Geometry: final body of the model. Coordinates: model frame, mm. A direction names the side the tool comes from. Coordinates: 2 decimals unless noted, no trailing zeros. Write each loop counter-clockwise with the first axis right and the second up, starting at its lowest first coordinate (ties: lowest second). Pieces come first, ordered by that corner, then holes. Notation, with made-up numbers: (26.5, -11.5) - (50.5, -11.5) arc R16 ccw to (50.5, 7.5) - close; hole circle Ø5 at (64, 88). An arc over 180 degrees is marked (long way). Answer as a JSON object with one key per item and string values. Group by question number.
Item 1: First-contact query: pin 1 Ø10 at (x, y) = (19.5, -27) entering from -Z; pin 2 Ø4 at (x, z) = (26, -11.5) entering from +Y; pin 3 Ø3.5 at (x, y) = (-1.5, -3) entering from -Z. Flat tips, straight axial feed; report the tip coordinate or a pass-through.
Item 2: Section B-B on x = 22. Return loops of the section in (y, z), and give its area (3 significant figures).
Item 3: Line query: line 1 along Y through (x, z) = (17, -10.5); line 2 along Z through (x, y) = (17, -31.2); line 3 along X through (y, z) = (-30.05, 6). Output: solid intervals per line, ascending. Write a range as from..to.
Item 4: Section A-A on z = -18. State how many separate pieces and enclosed holes the cut face has, and give its area (3 significant figures).
Item 5: Set-up query: faces 5 (the flat face through (0, -27, 4)), 6 (the cylindrical face through (43.53, -30.48, 0.18)), 7 (the flat face through (13, -19, -7)). Return all of +Z, -Z, +X, -X, +Y, -Y with unobstructed straight access to the full face (end or side cutting, diameter ignored); none if empty.
Item 6: Section D-D on y = -24. Return loops of the section in (x, z), and give its area (4 significant figures).
Item 7: Mould query, pull axis Z, two halves, no side actions, for faces 1 (the cylindrical face through (15.265, -30.479, 5.772)), 2 (the flat face through (22, -5, -3)), 3 (the flat face through (9, -16, -24)), 4 (the flat face through (11, -12, 10)). Classes: pulls with the +Z half, pulls with the -Z half, needs draft (parallel to the pull), parting line crosses it, or undercut.
```python
from build123d import *

# Parameters (mm, degrees)
SZKIC1_W                     = 12
SZKIC1_H                     = 18
SZKIC1_R                     = 1.75
DODANIE_WYCI_GNI_CIE1_DEPTH  = 5
SZKIC2_W                     = 12
SZKIC2_H                     = 36
SZKIC2_R                     = 1.75
DODANIE_WYCI_GNI_CIE2_DEPTH  = 5
SZKIC5_W                     = 34
SZKIC5_H                     = 4
DODANIE_WYCI_GNI_CIE5_DEPTH  = 38
SZKIC6_W                     = 7
SZKIC6_H                     = 34
DODANIE_WYCI_GNI_CIE6_DEPTH  = 18
SZKIC7_R                     = 1.75
WYTNIJ_WYCI_GNI_CIE1_DEPTH   = 4
WYTNIJ_WYCI_GNI_CIE2_DEPTH   = 4
ZAOKR_GLENIE1_R              = 5
SZKIC9_W                     = 5
SZKIC9_H                     = 18
DODANIE_WYCI_GNI_CIE7_DEPTH  = 12
DODANIE_WYCI_GNI_CIE8_DEPTH  = 18
SZKIC11_W                    = 4
SZKIC11_H                    = 34
DODANIE_WYCI_GNI_CIE9_DEPTH  = 2
SZKIC12_R                    = 1.75
SZKIC12_W                    = 4
SZKIC12_H                    = 34
DODANIE_WYCI_GNI_CIE10_DEPTH = 3
SFAZOWANIE1_SIZE             = 3
SFAZOWANIE2_SIZE             = 2
SZKIC13_W                    = 3
SZKIC13_H                    = 34
DODANIE_WYCI_GNI_CIE11_DEPTH = 14
SZKIC14_R                    = 1.75
WYTNIJ_WYCI_GNI_CIE3_DEPTH   = 3


with BuildPart() as part:
    # Szkic1 → Dodanie-wyciągnięcie1 (new body)
    with BuildSketch(Plane.XY):
        Rectangle(SZKIC1_W, SZKIC1_H)
        with Locations((-2, 5)):
            Circle(SZKIC1_R, mode=Mode.SUBTRACT)
        with Locations((2, -5)):
            Circle(SZKIC1_R, mode=Mode.SUBTRACT)
    extrude(amount=DODANIE_WYCI_GNI_CIE1_DEPTH)

    # Szkic2 → Dodanie-wyciągnięcie2 (add)
    with BuildSketch(Plane.XY.offset(5)):
        with Locations((0, -9)):
            Rectangle(SZKIC2_W, SZKIC2_H)
        with Locations((-2, 5)):
            Circle(SZKIC2_R, mode=Mode.SUBTRACT)
        with Locations((2, -5)):
            Circle(SZKIC2_R, mode=Mode.SUBTRACT)
    extrude(amount=DODANIE_WYCI_GNI_CIE2_DEPTH)

    # Szkic5 → Dodanie-wyciągnięcie5 (add)
    with BuildSketch(Plane(origin=(6, 0, 0), x_dir=(0, 0, -1), z_dir=(1, 0, 0))):
        with Locations((7, -7)):
            Rectangle(SZKIC5_W, SZKIC5_H)
    extrude(amount=DODANIE_WYCI_GNI_CIE5_DEPTH)

    # Szkic6 → Dodanie-wyciągnięcie6 (add)
    with BuildSketch(Plane.XZ.offset(9)):
        with Locations((9.5, -7)):
            Rectangle(SZKIC6_W, SZKIC6_H)
    extrude(amount=DODANIE_WYCI_GNI_CIE6_DEPTH)

    # Szkic7 → Wytnij-wyciągnięcie1 (cut)
    with BuildSketch(Plane(origin=(0, -5, 0), x_dir=(1, 0, 0), z_dir=(0, 1, 0))):
        with Locations(Location((17, -6, 0), (0, 0, 270))):
            Circle(SZKIC7_R)
        with Locations(Location((17, 18, 0), (0, 0, 270))):
            Circle(SZKIC7_R)
        with Locations(Location((38.7, -6, 0), (0, 0, 270))):
            Circle(SZKIC7_R)
    extrude(amount=-WYTNIJ_WYCI_GNI_CIE1_DEPTH, mode=Mode.SUBTRACT)

    # Szkic8 → Wytnij-wyciągnięcie2 (cut)
    with BuildSketch(Plane(origin=(0, -5, 0), x_dir=(1, 0, 0), z_dir=(0, 1, 0))):
        Polygon((44, 24), (16, 24), (44, 0), align=None)
    extrude(amount=-WYTNIJ_WYCI_GNI_CIE2_DEPTH, mode=Mode.SUBTRACT)

    # Zaokrąglenie1
    zaokr_glenie1_edges = [part.edges().sort_by_distance(p)[0] for p in [
        (44, -7, 10),
        (16, -7, -24),
        (44, -7, 0),
    ]]
    fillet(zaokr_glenie1_edges, radius=ZAOKR_GLENIE1_R)

    # Szkic9 → Dodanie-wyciągnięcie7 (add)
    with BuildSketch(Plane.ZY.offset(-6)):
        with Locations((2.5, -18)):
            Rectangle(SZKIC9_W, SZKIC9_H)
    extrude(amount=DODANIE_WYCI_GNI_CIE7_DEPTH)

    # Szkic10 → Dodanie-wyciągnięcie8 (add)
    with BuildSketch(Plane.XZ.offset(27)):
        Polygon((6, 0), (1, 0), (6, -5), align=None)
    extrude(amount=-DODANIE_WYCI_GNI_CIE8_DEPTH)

    # Szkic11 → Dodanie-wyciągnięcie9 (add)
    with BuildSketch(Plane.XZ.offset(27)):
        with Locations((11, -7)):
            Rectangle(SZKIC11_W, SZKIC11_H)
    extrude(amount=DODANIE_WYCI_GNI_CIE9_DEPTH)

    # Szkic12 → Dodanie-wyciągnięcie10 (add)
    # profile 1 of 2: a face of its own
    with BuildSketch(Plane.XZ.offset(29)):
        with BuildLine():
            Line((44, 2.299674612), (44, 5))
            ThreePointArc((44, 5), (42.535533906, 8.535533906), (39, 10))
            Line((39, 10), (13, 10))
            Line((13, 10), (13, -24))
            Line((13, -24), (14.150379619, -24))
            ThreePointArc((14.150379619, -24), (15.885110858, -23.689425075), (17.404336486, -22.796283012))
            Line((17.404336486, -22.796283012), (42.253956867, -1.496608399))
            ThreePointArc((42.253956867, -1.496608399), (43.542564492, 0.210390565), (44, 2.299674612))
        make_face()
        with Locations(Location((38.7, 6, 0), (0, 0, 90))):
            Circle(SZKIC12_R, mode=Mode.SUBTRACT)
        with Locations(Location((17, -18, 0), (0, 0, 90))):
            Circle(SZKIC12_R, mode=Mode.SUBTRACT)
        with Locations(Location((17, 6, 0), (0, 0, 90))):
            Circle(SZKIC12_R, mode=Mode.SUBTRACT)
    # profile 2 of 2: a face of its own
    with BuildSketch(Plane.XZ.offset(29)):
        with Locations((11, -7)):
            Rectangle(SZKIC12_W, SZKIC12_H)
    extrude(amount=DODANIE_WYCI_GNI_CIE10_DEPTH)

    # Sfazowanie1
    sfazowanie1_edges = [part.edges().sort_by_distance(p)[0] for p in [
        (9, -27, -7),
    ]]
    chamfer(sfazowanie1_edges, length=SFAZOWANIE1_SIZE)

    # Sfazowanie2
    sfazowanie2_edges = [part.edges().sort_by_distance(p)[0] for p in [
        (9, -32, -7),
    ]]
    chamfer(sfazowanie2_edges, length=SFAZOWANIE2_SIZE - 0.0001)  # a hair under: the kernel refuses the full size

    # Szkic13 → Dodanie-wyciągnięcie11 (add)
    with BuildSketch(Plane(origin=(0, -5, 0), x_dir=(1, 0, 0), z_dir=(0, 1, 0))):
        with Locations((7.5, 7)):
            Rectangle(SZKIC13_W, SZKIC13_H)
    extrude(amount=DODANIE_WYCI_GNI_CIE11_DEPTH)

    # Szkic14 → Wytnij-wyciągnięcie3 (cut)
    with BuildSketch(Plane(origin=(9, 0, 0), x_dir=(0, 0, -1), z_dir=(1, 0, 0))):
        with Locations((7, 1)):
            Circle(SZKIC14_R)
    extrude(amount=-WYTNIJ_WYCI_GNI_CIE3_DEPTH, mode=Mode.SUBTRACT)


solid = part.part
```
Checks:
{
 "1": {"pin 1": "z = -23.94", "pin 2": "y = -5", "pin 3": "z = 0"},
 "2": {"outline": "(-32, -18.86) - (-29, -18.86) - (-29, 10) - (-32, 10) - close; (-9, -18.86) - (-5, -18.86) - (-5, 10) - (-9, 10) - close", "area": "202 mm^2"},
 "3": {"line 1": "-32..-29, -9..-5", "line 2": "-23.11..-19.75, -16.25..4.25, 7.75..10", "line 3": "9.05..15.25, 18.75..36.95, 40.45..43.9"},
 "4": {"separate pieces": "3", "enclosed holes": "0", "area": "264 mm^2"},
 "5": {"face 5": "+Z, -Z, -X, -Y", "face 6": "-Z, +X, +Y, -Y", "face 7": "+Z, -Z, +X"},
 "6": {"outline": "(-6, 0) - (1, 0) - (6, -5) - (6, -24) - (13, -24) - (13, 10) - (-6, 10) - close", "area": "370.5 mm^2"},
 "7": {"face 1": "undercut", "face 2": "needs draft", "face 3": "pulls with the -Z half", "face 4": "pulls with the +Z half"}
}
